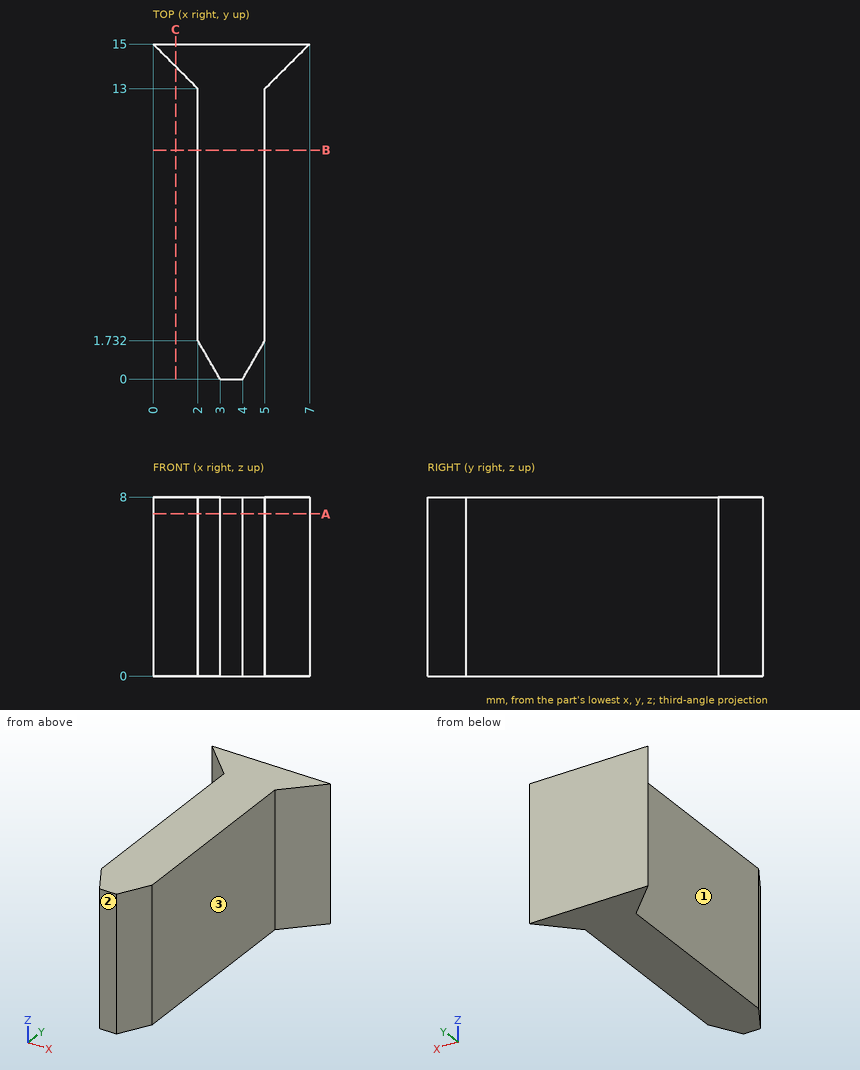
Input: dimensioned drawing with shaded views. Units: mm. Origin: part minimum x, y, z. A direction names the side the tool comes from. Coordinates: 2 decimals unless noted, no trailing zeros. Write each loop counter-clockwise with the first axis right and the second up, starting at its lowest first coordinate (ties: lowest second). Pieces come first, ordered by that corner, then holes. Notation, with made-up numbers: M 43.25,38.25 L 99.25,38.25 A28 ccw 99.25,60.25 Z; hole C -7,-32 d3. An arc over 180 degrees is marked long. Answer as a JSON object with one key per item and string values. Group by question number.
(1) Section A-A on z = 7.25. Output: boundary loops of the cut face in (x, y).
(2) Set-up query: the marked faces 1, 2 and 3. Return all of +Z, -Z, +X, -X, +Y, -Y with unobstructed straight access to the full face (end or side cutting, diameter ignored); none if empty.
(3) Contact query for flat-ended pins moving along their axis: P1, Ø4, axis at y = 6.5, z = 4, coming from the -X side; P2, Ø4, axis at y = 2, z = 2.5, coming from the +X side. Output: stop coordinate, or through.
(4) Section B-B on y = 10.25. Output: boundary loops of the cut face in (x, z).
(5) Ray query, line 1 along X through (y, z) = (6, 4.25); line 2 along Y through (x, z) = (2.75, 0.5); line 3 along Y through (x, z) = (6.25, 5.25). Return the intervals inside material, ascending. Write a range as [from, to].
(6) Section C-C on x = 1. Output: boundary loops of the cut face in (y, z).
Result set:
{
 "1": {"outline": "M 0,15 L 2,13 L 2,1.73 L 3,0 L 4,0 L 5,1.73 L 5,13 L 7,15 Z"},
 "2": {"face 1": "+Z, -Z, -X, -Y", "face 2": "+Z, -Z, +X, -X, -Y", "face 3": "+Z, -Z, +X, -Y"},
 "3": {"P1": "stops at x = 2", "P2": "stops at x = 5"},
 "4": {"outline": "M 2,0 L 5,0 L 5,8 L 2,8 Z"},
 "5": {"line 1": "x = [2, 5]", "line 2": "y = [0.43, 15]", "line 3": "y = [14.25, 15]"},
 "6": {"outline": "M 14,0 L 15,0 L 15,8 L 14,8 Z"}
}
